Can you work these out from the drawing? Everything is in mm from the part's minimum corner. A direction names the side the tool comes from. Give positions to 0.01 mm unless a question says otherwise; leave off trailing zeros. Write each loop counter-clockwise with the first axis right and the second up, starting at its lowest first coordinate (ties: lowest second). Pieces come first, ordered by that corner, then holes. Notation, with made-up numbers: (19.25, 68) - (49.25, 68) arc R7 ccw to (49.25, 78) - close; hole circle Ø3 at (-9, 38). An arc over 180 degrees is marked (long way). Answer in a Markdown table with one row per item.
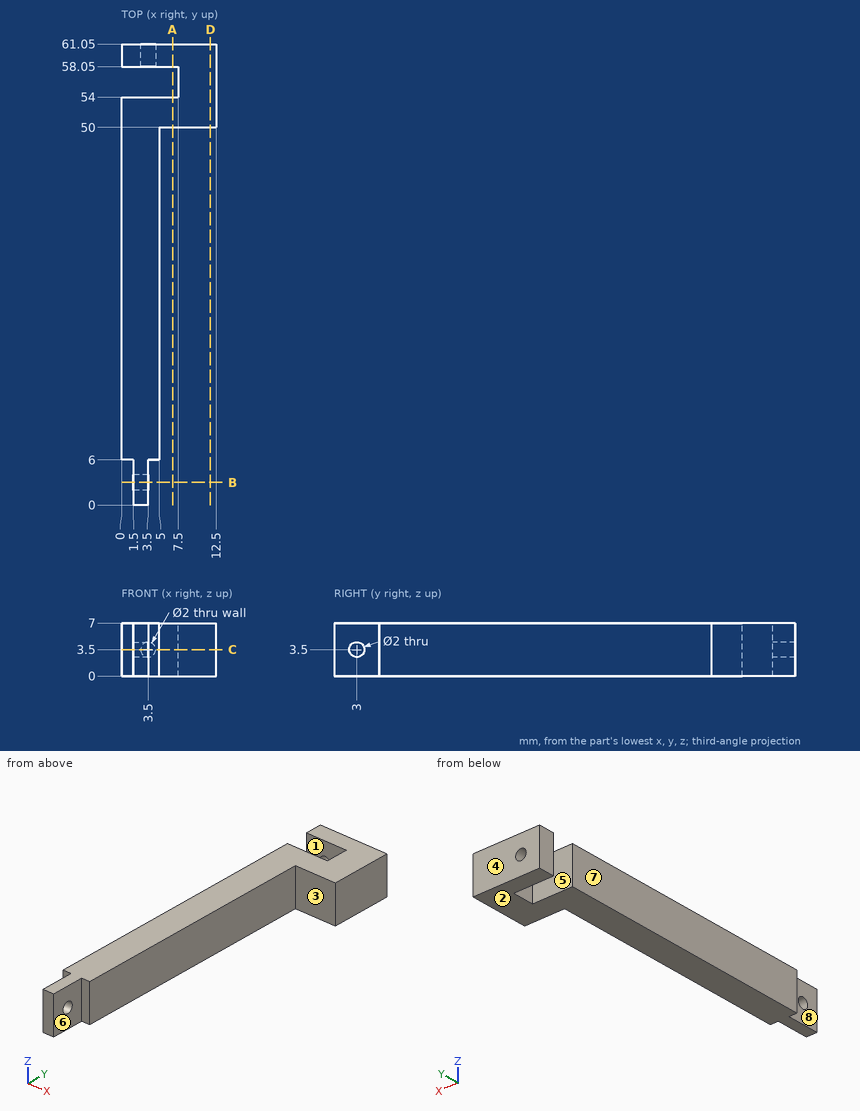
1) Imagine slicing it at D-D (x = 11.75). List the corners of the cut face in (y, z) for me.
Check values:
| item | result |
|---|---|
| outline | (50, 0) - (61.05, 0) - (61.05, 7) - (50, 7) - close |
2) Imagine slicing it at A-A (x = 6.75). List the corners of the cut face in (y, z) for me.
Check values:
| item | result |
|---|---|
| outline | (50, 0) - (54, 0) - (54, 7) - (50, 7) - close; (58.05, 0) - (61.05, 0) - (61.05, 7) - (58.05, 7) - close |
3) Imagine slicing it at C-C (z = 3.5). List the corners of the cut face in (x, y) for me.
Check values:
| item | result |
|---|---|
| outline | (0, 6) - (1.5, 6) - (1.5, 4) - (3.5, 4) - (3.5, 6) - (5, 6) - (5, 50) - (12.5, 50) - (12.5, 61.05) - (4.5, 61.05) - (4.5, 58.05) - (7.5, 58.05) - (7.5, 54) - (0, 54) - close; (0, 58.05) - (2.5, 58.05) - (2.5, 61.05) - (0, 61.05) - close; (1.5, 0) - (3.5, 0) - (3.5, 2) - (1.5, 2) - close |
4) Imagine slicing it at B-B (y = 3). List the corners of the cut face in (x, z) for me.
Check values:
| item | result |
|---|---|
| outline | (1.5, 0) - (3.5, 0) - (3.5, 2.5) - (1.5, 2.5) - close; (1.5, 4.5) - (3.5, 4.5) - (3.5, 7) - (1.5, 7) - close |
5) We'd pull the mould along Y, two halves only. Please class the marked faces 1, 2 and 3: +Y half, -Y half, draft (parallel to the pull), parting line (faces both ways), or undercut.
Check values:
| item | result |
|---|---|
| face 1 | undercut |
| face 2 | draft |
| face 3 | -Y half |
6) Will these pins go through, and if not, where does the flat tip stop? P1, Ø3, axis at y = 2, z = 5, coming from the -X side; P2, Ø1.2, axis at x = 0.5, z = 2.5, coming from the -Y side; P3, Ø2, axis at y = 55.5, z = 5, coming from the -X side.
Check values:
| item | result |
|---|---|
| P1 | stops at x = 1.5 |
| P2 | stops at y = 6 |
| P3 | stops at x = 7.5 |
7) If I drill on line 1 (Y direction, x = 2.4, z = 3.5); line 2 (Y direction, x = 7.25, z = 6.75); line 3 (Y direction, x = 2.8, z = 3.5), over which ranges is the centre line in solid material (lowest first)?
Check values:
| item | result |
|---|---|
| line 1 | y = 0 to 2, 4 to 54, 58.05 to 61.05 |
| line 2 | y = 50 to 54, 58.05 to 61.05 |
| line 3 | y = 0 to 2, 4 to 54 |
8) On a 3-axis mill with a long thin cutter (end or side, diameter ignored), from which of +Z, -Z, +X, -X, +Y, -Y can I reach the whole of each face in a straight line? I mean the marked faces 4, 5, 6, 7 and 8. Say none if no direction works.
Check values:
| item | result |
|---|---|
| face 4 | +Z, -Z, +X, -X, +Y |
| face 5 | +Z, -Z, -X |
| face 6 | +Z, -Z, +X, -Y |
| face 7 | +Z, -Z, -X, +Y, -Y |
| face 8 | +Z, -Z, -X, -Y |
